Input: dimensioned drawing with shaded views. Units: mm. Origin: part minimum x, y, z. Give positions to 0.01 mm unless a question says otherwise; leave off trailing zeros. Write each loop counter-clockwise with the first axis right and the second up, starting at its lowest first coordinate (ties: lowest second). Pieces come first, ordered by that corner, then holes. Notation, with made-up numbers: (-24.75, 7) -> (6.25, 7) arc R32 cw to (6.25, 43) -> close; hole circle Ø3 at (-4.5, 18.25). An arc over 180 degrees is marked (long way). Answer as a JSON object with one key per item and string values. Group by question number.
(1) Section query C-C on z = 2.25. Output: boundary loops of the cut face in (x, y).
(2) Section query B-B on y = 9. Output: boundary loops of the cut face in (x, z), plus the area to 3 significant figures.
(3) Section query A-A on x = 11.5. Output: boundary loops of the cut face in (y, z).
(4) Material intervals for probe 1 along Y at (x, z) = (120.5, 4.25); probe 2 along Z at (x, y) = (17, 7.5), sorted ascending.
(5) Contact query for flat-ended pins moving along their axis: pin 1 Ø4 at (x, z) = (41.5, 1.5) entering from -Y; pin 2 Ø10 at (x, y) = (99.5, 5.5) entering from -Z. Output: stop coordinate, or through.
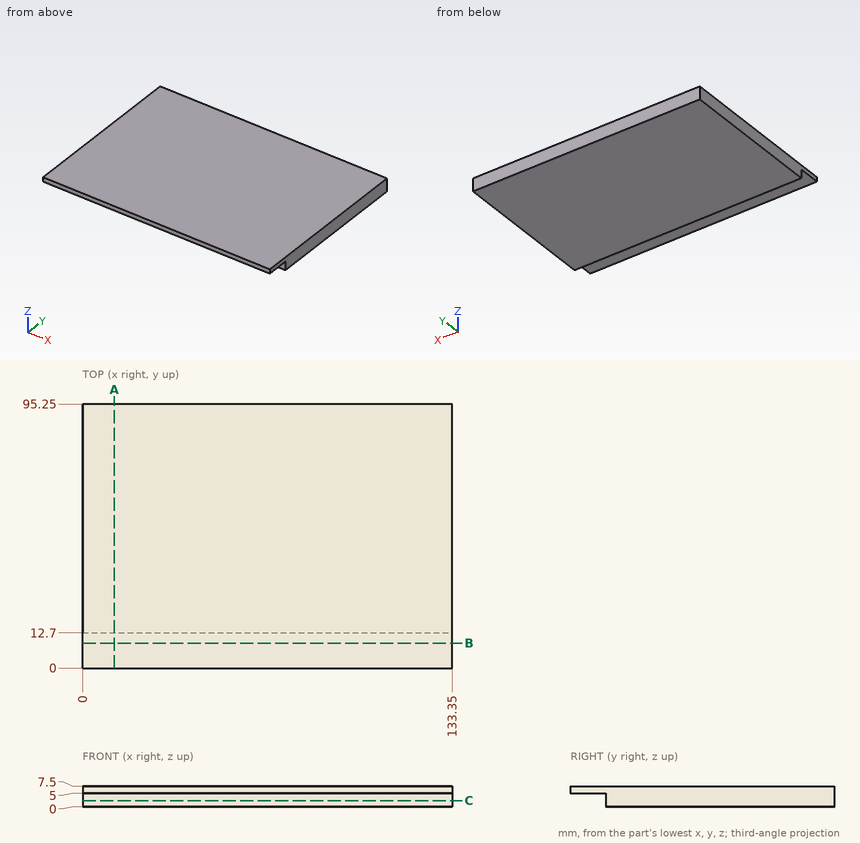
Answer list:
{
 "1": {"outline": "(0, 12.7) -> (133.35, 12.7) -> (133.35, 95.25) -> (0, 95.25) -> close"},
 "2": {"outline": "(0, 5) -> (133.35, 5) -> (133.35, 7.5) -> (0, 7.5) -> close", "area": "333 mm2"},
 "3": {"outline": "(0, 5) -> (12.7, 5) -> (12.7, 0) -> (95.25, 0) -> (95.25, 7.5) -> (0, 7.5) -> close"},
 "4": {"probe 1": "12.7 to 95.25", "probe 2": "5 to 7.5"},
 "5": {"pin 1": "y = 12.7", "pin 2": "z = 5"}
}
